Check sheet for the modelled part. Datum: model origin and axes. Units: mm. Coordinates: 2 decimals unless noted, no trailing zeros. Loops run counter-clockwise (first coordinate to the right, second up) from the corner with the lowest first, then second, coordinate; pieces in that order, holes last. Notation, with made-up numbers: M 37.25,8.5 L 41.25,8.5 A20 ccw 41.25,41.5 Z; hole C 33.25,10 d11. An arc over 180 degrees is marked long. Use CSV: the item, a comma, the result in double quotes. Start each with the question number.
(1) Section check C-C on x = 1.5. Record the cut outline in (y, z).
(2) Scan lines: line 1 (Z direction, x = 0.95, y = -15.5); line 2 (Y direction, x = 0.35, z = 13.5); line 3 (Y direction, x = 1.3, z = 14.5). Record each from-to range of solid material in increasing order.
(3) Section check A-A on z = 0. Record the cut outline in (x, y), and give its area (3 significant figures).
(4) Section check D-D on z = -15.5. Record the cut outline in (x, y).
(5) Draft check along Y on faces 1 (the flat face through (1, 0, -21.15)), 2 (the cylindrical face through (0.99, -2.38, -10.74)), 3 (the cylindrical face through (0.986, 16.538, 13.504)), 4 (the flat face through (1, -21.15, 0)). Enter one of: pulls with the +Y half, pulls with the -Y half, needs draft (parallel to the pull), parting line crosses it, or undercut.
(6) Section check B-B on y = -6. Record the cut outline in (x, z), and give its area (3 significant figures).
from build123d import *

# Parameters (mm, degrees)
F0_W     = 42.3
F0_H     = 42.3
F0_R     = 2.25
F0_R_2   = 11
F1_DEPTH = 2
F2_SIZE  = 5


with BuildPart() as f1:
    # F0 (on Right) → F1 (new body)
    with BuildSketch(Plane.YZ):
        Rectangle(F0_W, F0_H)
        with Locations((-15.5, -15.5)):
            Circle(F0_R, mode=Mode.SUBTRACT)
        with Locations((15.5, -15.5)):
            Circle(F0_R, mode=Mode.SUBTRACT)
        with Locations((-15.5, 15.5)):
            Circle(F0_R, mode=Mode.SUBTRACT)
        Circle(F0_R_2, mode=Mode.SUBTRACT)
        with Locations((15.5, 15.5)):
            Circle(F0_R, mode=Mode.SUBTRACT)
    extrude(amount=F1_DEPTH)

    # F2
    f2_edges = [f1.edges().sort_by_distance(p)[0] for p in [
        (1, -21.15, 21.15),
        (1, 21.15, 21.15),
        (1, -21.15, -21.15),
        (1, 21.15, -21.15),
    ]]
    chamfer(f2_edges, length=F2_SIZE)


solid = f1.part
Outcome:
1,outline,"M -21.15,-16.15 L -16.15,-21.15 L 16.15,-21.15 L 21.15,-16.15 L 21.15,16.15 L 16.15,21.15 L -16.15,21.15 L -21.15,16.15 Z; hole C -15.5,-15.5 d4.5; hole C -15.5,15.5 d4.5; hole C 0,0 d22; hole C 15.5,-15.5 d4.5; hole C 15.5,15.5 d4.5"
2,line 1,"z = -21.15 to -17.75, -13.25 to 13.25, 17.75 to 21.15"
2,line 2,"y = -21.15 to -16.53, -14.47 to 14.47, 16.53 to 21.15"
2,line 3,"y = -21.15 to -17.52, -13.48 to 13.48, 17.52 to 21.15"
3,outline,"M 0,-21.15 L 2,-21.15 L 2,-11 L 0,-11 Z; M 0,11 L 2,11 L 2,21.15 L 0,21.15 Z"
3,area,"40.6 mm²"
4,outline,"M 0,-21.15 L 2,-21.15 L 2,-17.75 L 0,-17.75 Z; M 0,-13.25 L 2,-13.25 L 2,13.25 L 0,13.25 Z; M 0,17.75 L 2,17.75 L 2,21.15 L 0,21.15 Z"
5,face 1,"needs draft"
5,face 2,"undercut"
5,face 3,"undercut"
5,face 4,"pulls with the -Y half"
6,outline,"M 0,-21.15 L 2,-21.15 L 2,-9.22 L 0,-9.22 Z; M 0,9.22 L 2,9.22 L 2,21.15 L 0,21.15 Z"
6,area,"47.7 mm²"
